```python
from build123d import *

# Parameters (mm, degrees)
F0_R     = 44.5
F0_R_2   = 1.5
F0_R_3   = 32
F1_DEPTH = 7
F2_DEPTH = 15
F0_R_4   = 2.5
F3_DEPTH = 5


with BuildPart() as f1:
    # F0 (on Top) → F1 (new body)
    with BuildSketch(Plane.XY):
        Circle(F0_R)
        with Locations((0, -41)):
            Circle(F0_R_2, mode=Mode.SUBTRACT)
        with Locations((-41, 0)):
            Circle(F0_R_2, mode=Mode.SUBTRACT)
        Circle(F0_R_3, mode=Mode.SUBTRACT)
        with Locations((41, 0)):
            Circle(F0_R_2, mode=Mode.SUBTRACT)
        with Locations((0, 41)):
            Circle(F0_R_2, mode=Mode.SUBTRACT)
    extrude(amount=F1_DEPTH)

    # F0 (on Top) → F2 (join)
    with BuildSketch(Plane.XY):
        with BuildLine():
            ThreePointArc((36.2253641288, -29.1542963169), (43.8561821867, -15.455914208), (46.5, 0))
            ThreePointArc((46.5, 0), (43.8561821867, 15.455914208), (36.2253641288, 29.1542963169))
            ThreePointArc((36.2253641288, 29.1542963169), (32.8804653252, 32.8804653252), (29.1542963169, 36.2253641288))
            ThreePointArc((29.1542963169, 36.2253641288), (0, 46.5), (-29.1542963169, 36.2253641288))
            ThreePointArc((-29.1542963169, 36.2253641288), (-32.8804653252, 32.8804653252), (-36.2253641288, 29.1542963169))
            ThreePointArc((-36.2253641288, 29.1542963169), (-46.5, 0), (-36.2253641288, -29.1542963169))
            ThreePointArc((-36.2253641288, -29.1542963169), (-32.8804653252, -32.8804653252), (-29.1542963169, -36.2253641288))
            ThreePointArc((-29.1542963169, -36.2253641288), (0, -46.5), (29.1542963169, -36.2253641288))
            ThreePointArc((29.1542963169, -36.2253641288), (32.8804653252, -32.8804653252), (36.2253641288, -29.1542963169))
        make_face()
        Circle(F0_R, mode=Mode.SUBTRACT)
        Circle(F0_R_3)
    extrude(amount=F2_DEPTH)

    # F0 (on Top) → F3 (join)
    with BuildSketch(Plane.XY):
        with BuildLine():
            Line((-37.8302127935, -44.9012806053), (-29.1542963169, -36.2253641288))
            ThreePointArc((-29.1542963169, -36.2253641288), (-32.8804653252, -32.8804653252), (-36.2253641288, -29.1542963169))
            Line((-36.2253641288, -29.1542963169), (-44.9012806053, -37.8302127935))
            Line((-44.9012806053, -37.8302127935), (-37.8302127935, -44.9012806053))
        make_face()
        with Locations((-37.8302127935, -37.8302127935)):
            Circle(F0_R_4, mode=Mode.SUBTRACT)
        with BuildLine():
            ThreePointArc((-36.2253641288, 29.1542963169), (-32.8804653252, 32.8804653252), (-29.1542963169, 36.2253641288))
            Line((-29.1542963169, 36.2253641288), (-37.8302127935, 44.9012806053))
            Line((-37.8302127935, 44.9012806053), (-44.9012806053, 37.8302127935))
            Line((-44.9012806053, 37.8302127935), (-36.2253641288, 29.1542963169))
        make_face()
        with Locations((-37.8302127935, 37.8302127935)):
            Circle(F0_R_4, mode=Mode.SUBTRACT)
        with BuildLine():
            ThreePointArc((29.1542963169, 36.2253641288), (32.8804653252, 32.8804653252), (36.2253641288, 29.1542963169))
            Line((36.2253641288, 29.1542963169), (44.9012806053, 37.8302127935))
            Line((44.9012806053, 37.8302127935), (37.8302127935, 44.9012806053))
            Line((37.8302127935, 44.9012806053), (29.1542963169, 36.2253641288))
        make_face()
        with Locations((37.8302127935, 37.8302127935)):
            Circle(F0_R_4, mode=Mode.SUBTRACT)
        with BuildLine():
            Line((44.9012806053, -37.8302127935), (36.2253641288, -29.1542963169))
            ThreePointArc((36.2253641288, -29.1542963169), (32.8804653252, -32.8804653252), (29.1542963169, -36.2253641288))
            Line((29.1542963169, -36.2253641288), (37.8302127935, -44.9012806053))
            Line((37.8302127935, -44.9012806053), (44.9012806053, -37.8302127935))
        make_face()
        with Locations((37.8302127935, -37.8302127935)):
            Circle(F0_R_4, mode=Mode.SUBTRACT)
    extrude(amount=F3_DEPTH)


solid = f1.part
```
CAD build for the part. Positions are in the model's coordinates, mm. A direction names the side the tool comes from. Round coordinates to 2 decimals unless told otherwise and drop trailing zeros. Order: outer loops, then holes, each group sorted by start corner. A loop starts at its lowest first (then second) coordinate and runs counter-clockwise, first axis right, second up.
Q1. Which spindle directions (+Z, -Z, +X, -X, +Y, -Y) get a long thin tool onto all of the face, cutting with end or side? Do faces 5 (the flat face through (-35, 37, 5)), 6 (the flat face through (40.5, 33.43, 2.46)), 7 (the flat face through (33.55, 40.62, 2.46)), 8 (the cylindrical face through (-6.94, -31.24, 10.94)), 9 (the flat face through (-35, -37, 5)). Say none if no direction does.
Q2. Slice it at C-C (y = -17.5). Write the cut outline in (x, z), and give its area (3 significant figures).
Q3. Two-plate mould, pull along X, no slides. Class faces 1 (the flat face through (0, -33, 7)), 2 (the flat face through (-41.316, 41.415, 2.465)), 3 (the flat face through (40.62, -33.55, 2.46)), 4 (the cylindrical face through (-35.52, 36.87, 2.46)): pulls with the +X half, pulls with the -X half, needs draft (parallel to the pull), parting line crosses it, or undercut.
Q4. Wall check: L1, parallel to X at y = -39, z = 1.5; L2, parallel to Y at x = 25.5, z = 13.75; L3, parallel to X at y = -14, z = 7.25. Give the ranges that are in metal, low to high.
Q5. Slice it at D-D (y = 18.5). Write the cut outline in (x, z).
Q6. Slice it at A-A (z = 13.5). Write the cut outline in (x, y).
Q7. Slice it at B-B (x = 0). Write the cut outline in (y, z), and give its area (3 significant figures).
Q8. Drop flat-ended pins along their axis: pin 1 (1 mm diameter, centred on x = 19.5, z = 12.5, fed in from -Y); pin 2 (4.5 mm diameter, centred on x = 40.5, y = 39.5, fed in from +Z); pin 3 (8 mm diameter, centred on y = 25, z = 11, fed in from -X). Give the stop position or say it passes through.
Results below:
1. face 5: +Z, -X, +Y
1. face 6: +Z, -Z, +X
1. face 7: +Z, -Z, +Y
1. face 8: +Z
1. face 9: +Z, -X, -Y
2. outline: (-43.08, 0) - (43.08, 0) - (43.08, 15) - (40.91, 15) - (40.91, 7) - (26.79, 7) - (26.79, 15) - (-26.79, 15) - (-26.79, 7) - (-40.91, 7) - (-40.91, 15) - (-43.08, 15) - close
2. area: 1,070 mm2
3. face 1: undercut
3. face 2: pulls with the -X half
3. face 3: pulls with the +X half
3. face 4: undercut
4. L1: x = -43.73 to -40.04, -35.62 to -31.93, -25.32 to 25.32, 31.93 to 35.62, 40.04 to 43.73
4. L2: y = -38.88 to -36.47, -19.33 to 19.33, 36.47 to 38.88
4. L3: x = -44.34 to -42.24, -28.77 to 28.77, 42.24 to 44.34
5. outline: (-42.66, 0) - (42.66, 0) - (42.66, 15) - (40.47, 15) - (40.47, 7) - (26.11, 7) - (26.11, 15) - (-26.11, 15) - (-26.11, 7) - (-40.47, 7) - (-40.47, 15) - (-42.66, 15) - close
6. outline: circle Ø93 at (0, 0); circle Ø64 at (0, 0); hole circle Ø89 at (0, 0)
7. outline: (-46.5, 0) - (-42.5, 0) - (-42.5, 7) - (-44.5, 7) - (-44.5, 15) - (-46.5, 15) - close; (-39.5, 0) - (39.5, 0) - (39.5, 7) - (32, 7) - (32, 15) - (-32, 15) - (-32, 7) - (-39.5, 7) - close; (42.5, 0) - (46.5, 0) - (46.5, 15) - (44.5, 15) - (44.5, 7) - (42.5, 7) - close
7. area: 1,150 mm2
8. pin 1: stops at y = -42.44
8. pin 2: stops at z = 5
8. pin 3: stops at x = -41.49
